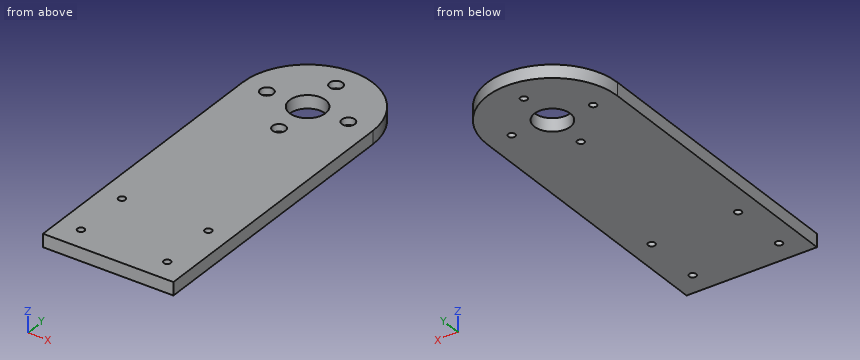
from build123d import *

# Parameters (mm, degrees)
SKETCH1_R                                           = 8
BOSS_EXTRUDE1_DEPTH                                 = 8
CBORE_FOR_M4_HEX_SOCKET_HEAD_CAP_SCREW2_D           = 4.3
CBORE_FOR_M4_HEX_SOCKET_HEAD_CAP_SCREW2_CBORE_D     = 8
CBORE_FOR_M4_HEX_SOCKET_HEAD_CAP_SCREW2_CBORE_DEPTH = 4.4
F_20_0MM_TRANSITIONAL_DOWEL_HOLE1_D                 = 22
M4_CLEARANCE_HOLE2_D                                = 4.3


with BuildPart() as part:
    # Sketch1 → Boss-Extrude1 (new body)
    with BuildSketch(Plane.XY):
        with BuildLine():
            Line((0, 0), (-80, 0))
            Line((-80, 0), (-80, 175))
            ThreePointArc((-80, 175), (-40, 215), (0, 175))
            Line((0, 175), (0, 0))
        make_face()
        with Locations((-40, 175)):
            Circle(SKETCH1_R, mode=Mode.SUBTRACT)
    extrude(amount=BOSS_EXTRUDE1_DEPTH)

    # CBORE for M4 Hex Socket Head Cap Screw2 (through all)
    with Locations(Plane.XY.offset(8)):
        with Locations((-40, 200), (-15, 175), (-40, 150), (-65, 175)):
            CounterBoreHole(CBORE_FOR_M4_HEX_SOCKET_HEAD_CAP_SCREW2_D / 2, CBORE_FOR_M4_HEX_SOCKET_HEAD_CAP_SCREW2_CBORE_D / 2, CBORE_FOR_M4_HEX_SOCKET_HEAD_CAP_SCREW2_CBORE_DEPTH)

    # Ø20.0mm Transitional Dowel Hole1 (through all)
    with Locations(Plane.XY.offset(8)):
        with Locations((-40, 175)):
            Hole(F_20_0MM_TRANSITIONAL_DOWEL_HOLE1_D / 2)

    # M4 Clearance Hole2 (through all)
    with Locations(Plane.XY.offset(8)):
        with Locations((-66.5, 50), (-13.5, 14), (-66.5, 14), (-13.5, 50)):
            Hole(M4_CLEARANCE_HOLE2_D / 2)


solid = part.part
Could you check a few things on this model? Use its own coordinates, in mm. Give positions to 0.01 mm unless a question says otherwise; leave off trailing zeros. Write each loop counter-clockwise with the first axis right and the second up, starting at its lowest first coordinate (ties: lowest second). Pieces come first, ordered by that corner, then holes. Notation, with made-up numbers: (87.25, 37.25) -> (136.25, 37.25) arc R20 cw to (136.25, 60.25) -> close; hole circle Ø5 at (-24.5, 11.25). An arc over 180 degrees is marked (long way). Write each question's results on one line, items separated by ' | '. Start each with the question number.
Q1. I'm going to push flat-ended pins straight in: pin 1 Ø5 at (x, y) = (-41, 109.5) entering from -Z; pin 2 Ø4 at (x, y) = (-15.5, 173.5) entering from +Z. Where does each tip first touch, or does it pass through?
Q2. Suppose I cut it at B-B, the plane x = -40. List the corners of the cut face in (y, z) for me, and give its area (3 significant figures).
Q3. Suppose I cut it at C-C, the plane z = 1.75. State how many separate pieces and enclosed holes the cut face has, and give its area (3 significant figures).
Q4. Suppose I cut it at A-A, the plane y = 14. List the corners of the cut face in (x, z) for me.
Q5. Suppose I cut it at D-D, the plane y = 150. List the corners of the cut face in (x, z) for me.
Q6. I need wall thicknesses on probe 1 along Y at (x, z) = (-40, 5.6); probe 2 along Y at (x, z) = (-15, 2.5); probe 3 along Y at (x, z) = (-31, 3.5). Which ranges of each line are inside material? Lowest first, please.
Outcome:
1) pin 1: z = 0 | pin 2: z = 3.6
2) outline: (0, 0) -> (147.85, 0) -> (147.85, 3.6) -> (146, 3.6) -> (146, 8) -> (0, 8) -> close; (152.15, 0) -> (164, 0) -> (164, 8) -> (154, 8) -> (154, 3.6) -> (152.15, 3.6) -> close; (186, 0) -> (197.85, 0) -> (197.85, 3.6) -> (196, 3.6) -> (196, 8) -> (186, 8) -> close; (202.15, 0) -> (215, 0) -> (215, 8) -> (204, 8) -> (204, 3.6) -> (202.15, 3.6) -> close | area: 1,440 mm2
3) separate pieces: 1 | enclosed holes: 9 | area: 16,000 mm2
4) outline: (-80, 0) -> (-68.65, 0) -> (-68.65, 8) -> (-80, 8) -> close; (-64.35, 0) -> (-15.65, 0) -> (-15.65, 8) -> (-64.35, 8) -> close; (-11.35, 0) -> (0, 0) -> (0, 8) -> (-11.35, 8) -> close
5) outline: (-80, 0) -> (-42.15, 0) -> (-42.15, 3.6) -> (-44, 3.6) -> (-44, 8) -> (-80, 8) -> close; (-37.85, 0) -> (0, 0) -> (0, 8) -> (-36, 8) -> (-36, 3.6) -> (-37.85, 3.6) -> close
6) probe 1: 0 to 146, 154 to 164, 186 to 196, 204 to 215 | probe 2: 0 to 12.46, 15.54 to 48.46, 51.54 to 172.85, 177.15 to 206.22 | probe 3: 0 to 168.68, 181.32 to 213.97
